Verification items for the finished model (mm, model axes). Face numbers are marked on the shaded views. A direction names the side the tool comes from. Round coordinates to 2 decimals unless told otherwise and drop trailing zeros. Order: outer loops, then holes, each group sorted by start corner. A loop starts at its lowest first (then second) coordinate and runs counter-clockwise, first axis right, second up. Notation, with made-up numbers: (84.25, 53.5) -> (143.25, 53.5) arc R15 cw to (143.25, 77.5) -> close; hole circle Ø8 at (-27, 65.5). An arc over 180 degrees is marked (long way). Put each result on its own line as item: value.
```python
from build123d import *

# Parameters (mm, degrees)
F0_R          = 12.7
F1_DEPTH      = 44.45
F2_R          = 7.9375
F3_DEPTH      = 247.65
F4_R          = 6.35
F5_DEPTH      = 17.78
F6_W          = 0.8584746265
F6_H          = 1.4799516648
F8_R          = 4.953
F9_DEPTH      = 25.4
F9_DEPTH_BACK = 25.4


with BuildPart() as f1:
    # F0 (on Front) → F1 (new body)
    with BuildSketch(Plane.XZ):
        Circle(F0_R)
    extrude(amount=-F1_DEPTH)

    # F2 (on face) → F3 (join)
    with BuildSketch(Plane.XZ):
        Circle(F2_R)
    extrude(amount=F3_DEPTH)

    # F4 (on face) → F5 (join)
    with BuildSketch(Plane.XZ.offset(247.65)):
        Circle(F4_R)
    extrude(amount=F5_DEPTH)

    # F6 (on Right) → F7 (revolve, cut)
    with BuildSketch(Plane.YZ):
        with Locations((-262.4607626867, 6.4914319664)):
            Rectangle(F6_W, F6_H)
    revolve(axis=Axis((0, -260.4791074991, 0), (0, 1, 0)), mode=Mode.SUBTRACT)

    # F8 (on Top) → F9 (cut, two sides)
    with BuildSketch(Plane.XY) as f9_sk:
        with Locations((0, 31.75)):
            Circle(F8_R)
    extrude(amount=-F9_DEPTH, mode=Mode.SUBTRACT)
    extrude(f9_sk.sketch, amount=F9_DEPTH_BACK, mode=Mode.SUBTRACT)


solid = f1.part
```
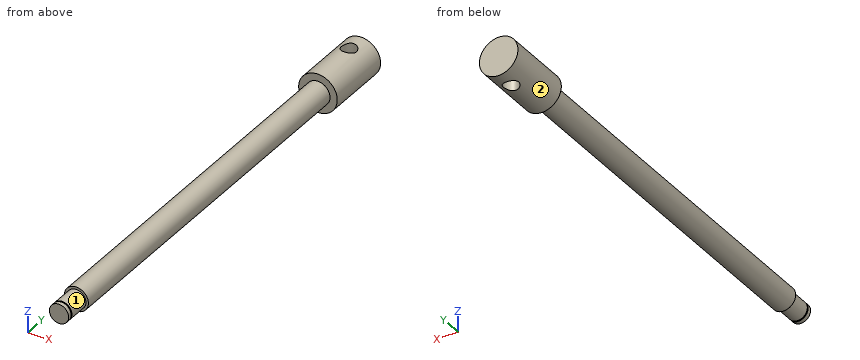
Item 1: Sectioned sample at B-B, the plane y = 31.75. Record the boundary of the cut face in (x, z).
Geometry check:
outline: (-4.95, -11.69) -> (-4.95, 11.69) arc R12.7 ccw to start; (4.95, -11.69) arc R12.7 ccw to (4.95, 11.69) -> close
Item 2: Material ranges on line 1 along Y through (x, z) = (0, -8.5); line 2 along X through (y, z) = (31.75, -5); line 3 along Y through (x, z) = (0, -7.75), recorded low to high.
Geometry check:
line 1: 0 to 26.8, 36.7 to 44.45
line 2: -11.67 to -4.95, 4.95 to 11.67
line 3: -247.65 to 26.8, 36.7 to 44.45
Item 3: Sectioned sample at A-A, the plane x = 0. Record the boundary of the cut face in (y, z), then the cut area to 3 significant figures.
Geometry check:
outline: (-265.43, -6.35) -> (-262.89, -6.35) -> (-262.89, -5.75) -> (-262.03, -5.75) -> (-262.03, -6.35) -> (-247.65, -6.35) -> (-247.65, -7.94) -> (0, -7.94) -> (0, -12.7) -> (26.8, -12.7) -> (26.8, 12.7) -> (0, 12.7) -> (0, 7.94) -> (-247.65, 7.94) -> (-247.65, 6.35) -> (-262.03, 6.35) -> (-262.03, 5.75) -> (-262.89, 5.75) -> (-262.89, 6.35) -> (-265.43, 6.35) -> close; (36.7, -12.7) -> (44.45, -12.7) -> (44.45, 12.7) -> (36.7, 12.7) -> close
area: 5,030 mm2
Item 4: Sectioned sample at C-C, the plane y = -180. Record the boundary of the cut face in (x, z) (1 decimal), then the cut area to 3 significant figures.
Geometry check:
outline: circle Ø15.9 at (0, 0)
area: 198 mm2
Item 5: Tool access check on the marked faces 1 and 2. Record the directions out of +Z, -Z, +X, -X, +Y, -Y that give a thin tool (end or side, any length) a straight path to the whole face; none if there is none.
Geometry check:
face 1: -Y
face 2: +Y, -Y
Item 6: Depth check by flat-ended pin: pin 1 Ø8 at (y, z) = (-232.5, 0.5) entering from +X; pin 2 Ø3 at (y, z) = (-102.5, -7.5) entering from -X; pin 3 Ø12 at (y, z) = (-62.5, -6.5) entering from -X; pin 4 Ø9 at (x, y) = (0, 31.75) entering from -Z. Enter the tip coordinate at first touch or a pass-through.
Geometry check:
pin 1: x = 7.94
pin 2: x = -5.2
pin 3: x = -7.92
pin 4: through
